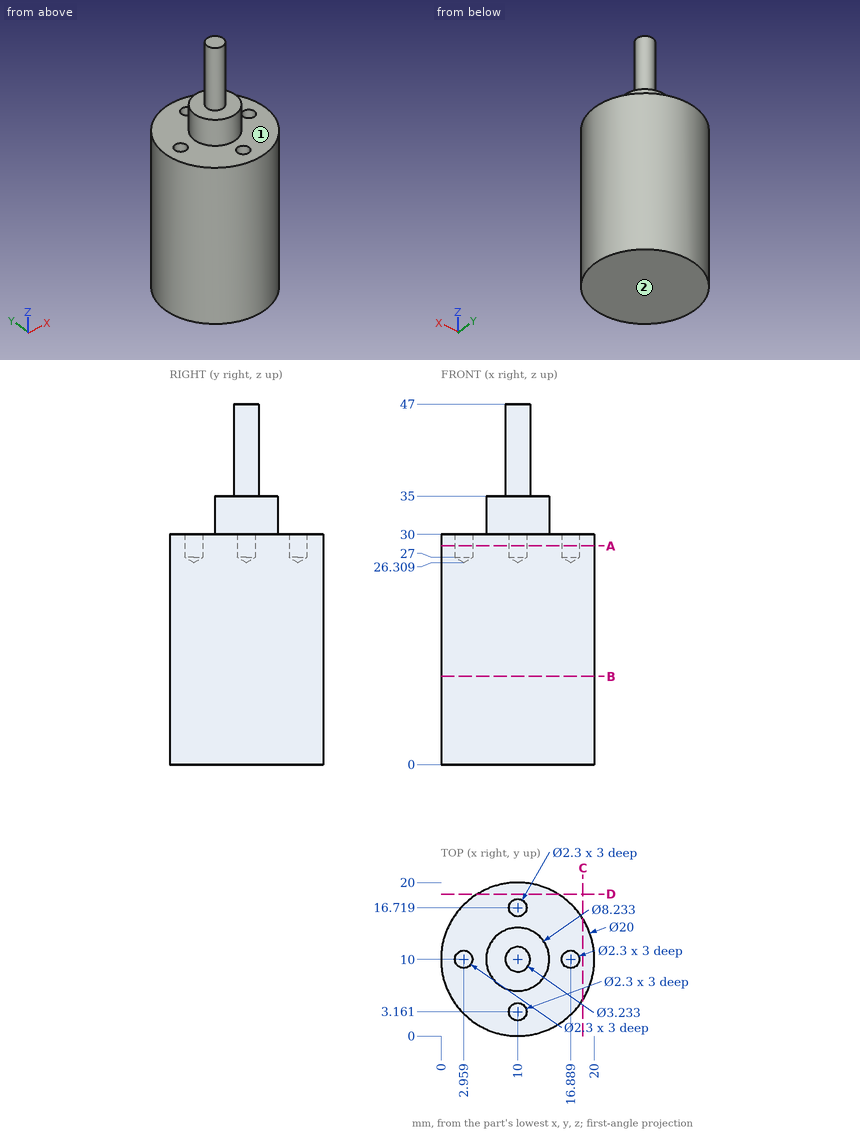
Part print with two shaded views. Sizes in mm from the minimum x, y, z corner. A direction names the side the tool comes from. Coordinates: 2 decimals unless noted, no trailing zeros. Write each loop counter-clockwise with the first axis right and the second up, starting at its lowest first coordinate (ties: lowest second). Pieces come first, ordered by that corner, then holes. Notation, with made-up numbers: (17, -2.5) -> (31, -2.5) arc R13 cw to (31, 13.5) -> close; hole circle Ø9 at (87.5, 29). An arc over 180 degrees is marked (long way). Return JSON: item names as keys, results as strings. Group by question number.
Q1. Flat gauge pins, fed straight in: pin 1 (2 mm diameter, centred on x = 16, z = 13.5, fed in from -Y); pin 2 (3 mm diameter, centred on x = 17, y = 14, fed in from -Z); pin 3 (3.5 mm diameter, centred on x = 10, y = 16.72, fed in from +Z); pin 4 (3 mm diameter, centred on x = 12, y = 13.5, fed in from +Z). Where does each tip first touch, or does it go through?
Q2. Drill centre lines: line 1 (Z direction, x = 5, y = 6.75); line 2 (Z direction, x = 12.5, y = 12.5); line 3 (X direction, y = 14.75, z = 5.5). Where is each one in solid material? Low to high.
Q3. Which spindle directions (+Z, -Z, +X, -X, +Y, -Y) get a long thin tool onto all of the face, cutting with end or side? Do the marked faces 1 and 2. Say none if no direction does.
Q4. Cut at A-A, the plane z = 28.5. Give the cut face in (x, y).
Q5. Cut at B-B, the plane z = 11.5. Give the cut face in (x, y), then the cut area to 3 significant figures.
Q6. Cut at C-C, the plane x = 18.5. Give the cut face in (y, z).
Returned:
{
 "1": {"pin 1": "stops at y = 1.34", "pin 2": "stops at z = 0", "pin 3": "stops at z = 30", "pin 4": "stops at z = 35"},
 "2": {"line 1": "z = 0 to 30", "line 2": "z = 0 to 35", "line 3": "x = 1.2 to 18.8"},
 "3": {"face 1": "+Z", "face 2": "-Z, +X, -X, +Y, -Y"},
 "4": {"outline": "circle Ø20 at (10, 10); hole circle Ø2.3 at (2.96, 10); hole circle Ø2.3 at (10, 3.16); hole circle Ø2.3 at (10, 16.72); hole circle Ø2.3 at (16.89, 10)"},
 "5": {"outline": "circle Ø20 at (10, 10)", "area": "314 mm2"},
 "6": {"outline": "(4.73, 0) -> (15.27, 0) -> (15.27, 30) -> (4.73, 30) -> close"}
}
